The listing builds one solid part. Answer for the finished solid, in the listing's coordinates (mm). A direction names the side the tool comes from. Give positions to 0.01 mm unless a question says otherwise; leave off trailing zeros. Write each loop counter-clockwise with the first axis right and the second up, starting at its lowest first coordinate (ties: lowest second). Pieces come first, ordered by that corner, then holes. Notation, with made-up numbers: M 17,38.5 L 72,38.5 A13 cw 72,62.5 Z; hole C -6.5,-1.5 d5. An arc over 180 degrees is marked long. Answer as a JSON object with one key per item and string values.
Autodesk Inventor part; units mm, degrees
ref_plane "YZ Plane" through (0, 0, 0) normal (1, 0, 0) x (0, 1, 0)
ref_plane "XZ Plane" through (0, 0, 0) normal (0, 1, 0) x (-1, 0, 0)
ref_plane "XY Plane" through (0, 0, 0) normal (0, 0, 1) x (1, 0, 0)
sketch "Sketch1" plane through (0, 0, 0) normal (0, 0, 1) x (1, 0, 0)
  line L0 (-13, 23) -> (13, 23)
  line L1 (15, 21) -> (15, -23)
  line L2 (15, -23) -> (-15, -23)
  line L3 (-15, -23) -> (-15, 21)
  line L4 (-15, 23) -> (15, -23) construction
  line L5 (15, 23) -> (-15, -23) construction
  line L6 (-13, 23) -> (-15, 21)
  line L7 (13, 23) -> (15, 21)
  circle A0 centre (-10, 18.5) radius 1.6
  circle A1 centre (10, 18.5) radius 1.6
  line L8 (10, 18.5) -> (-10, 18.5) construction
  point P0 (0, 0)
  point P1 (0, 18.5)
  point P2 (0, 0)
  dimension "d0" = 30
  dimension "d1" = 46
  dimension "d2" = 2
  dimension "d3" = 2
  dimension "d4" = 2
  dimension "d5" = 2
  dimension "d6" = 3.2
  dimension "d7" = 20
  dimension "d8" = 4.5
extrude "Extrusion1" add sketch "Sketch1" along normal blind 1.6
sketch "Sketch2" plane through (0, 0, 1.6) normal (0, 0, 1) x (1, 0, 0)
  line L0 (10.9, -19) -> (9.1, -19)
  line L1 (9.1, -19) -> (9.1, -4.2)
  line L2 (9.1, -4.2) -> (10.9, -4.2)
  line L3 (10.9, -4.2) -> (10.9, -19)
  line L4 (0.9, -19) -> (-0.9, -19)
  line L5 (-0.9, -19) -> (-0.9, -4.2)
  line L6 (-0.9, -4.2) -> (0.9, -4.2)
  line L7 (0.9, -4.2) -> (0.9, -19)
  line L8 (-9.1, -19) -> (-10.9, -19)
  line L9 (-10.9, -19) -> (-10.9, -4.2)
  line L10 (-10.9, -4.2) -> (-9.1, -4.2)
  line L11 (-9.1, -4.2) -> (-9.1, -19)
  line L12 (-15, 21) -> (-15, -23)
  line L13 (-15, -23) -> (15, -23)
  line L14 (15, -23) -> (15, 21)
  line L15 (15, 21) -> (13, 23)
  line L16 (13, 23) -> (-13, 23)
  line L17 (-13, 23) -> (-15, 21)
  circle A0 centre (10, 18.5) radius 1.6
  circle A1 centre (-10, 18.5) radius 1.6
  line L18 (-0.9, -4.2) -> (0.9, -19) construction
  line L19 (0.9, -4.2) -> (-0.9, -19) construction
  line L20 (10.9, -4.2) -> (9.1, -19) construction
  line L21 (9.1, -4.2) -> (10.9, -19) construction
  line L22 (-10.9, -4.2) -> (-9.1, -19) construction
  line L23 (-9.1, -4.2) -> (-10.9, -19) construction
  point P0 (0, 0)
  point P1 (0, -11.6)
  dimension "d11" = 1.8
  dimension "d12" = 14.8
  dimension "d13" = 4
  dimension "d14" = 8.2
  dimension "d15" = 8.2
extrude "Extrusion2" add sketch "Sketch2" along normal blind 18.2 contours L0 L1 L2 L3 | L4 L5 L6 L7 | L8 L9 L10 L11
fillet "Fillet1" radius 1 6 edges at (-10, -19, 19.8) (-10, -4.2, 19.8) (0, -4.2, 19.8) (0, -19, 19.8) (10, -19, 19.8) (10, -4.2, 19.8)
sketch "Sketch3" plane through (9.1, -19, 1.6) normal (-1, 0, 0) x (0, 0, 1)
  arc A0 (18.2, 13.8) -> (17.2, 14.8) centre (17.2, 13.8) ccw
  line L0 (0, 14.8) -> (17.2, 14.8)
  line L1 (0, 0) -> (0, 14.8)
  line L2 (0, 0) -> (17.2, 0)
  arc A1 (17.2, 0) -> (18.2, 1) centre (17.2, 1) ccw
  line L3 (18.2, 13.8) -> (18.2, 1)
  line L4 (0, 0) -> (0, 14.8)
  line L5 (10, 13.4) -> (0, 13.4)
  line L6 (0, 13.4) -> (0, 1.4)
  line L7 (0, 1.4) -> (10, 1.4)
  line L8 (10, 1.4) -> (10, 13.4)
  line L9 (10, 13.4) -> (0, 1.4) construction
  line L10 (0, 13.4) -> (10, 1.4) construction
  point P0 (-1.6, 19)
  point P1 (5, 7.4)
  point P2 (5, 7.4)
  point P3 (18.2, 7.4)
  point P4 (0, 13.4)
  point P5 (0, 1.4)
  dimension "d19" = 10
  dimension "d20" = 12
extrude "Extrusion3" add sketch "Sketch3" along normal up to surface (18.2 mm away) contours L5 L8 L7 L1
sketch "Sketch4" plane through (0, 0, 1.6) normal (0, 0, 1) x (1, 0, 0)
  circle A0 centre (-10, 18.5) radius 1.6
  circle A1 centre (10, 18.5) radius 1.6
  line L0 (-15, 21) -> (-15, -23)
  line L1 (-15, -23) -> (15, -23)
  line L2 (15, -23) -> (15, 21)
  line L3 (15, 21) -> (13, 23)
  line L4 (13, 23) -> (-13, 23)
  line L5 (-13, 23) -> (-15, 21)
  line L6 (-0.9, -17.6) -> (-9.1, -17.6)
  line L7 (-9.1, -17.6) -> (-9.1, -19)
  line L8 (-9.1, -19) -> (-10.9, -19)
  line L9 (-10.9, -19) -> (-10.9, -4.2)
  line L10 (-10.9, -4.2) -> (-9.1, -4.2)
  line L11 (-9.1, -4.2) -> (-9.1, -5.6)
  line L12 (-9.1, -5.6) -> (-0.9, -5.6)
  line L13 (-0.9, -5.6) -> (-0.9, -4.2)
  line L14 (-0.9, -4.2) -> (0.9, -4.2)
  line L15 (0.9, -4.2) -> (0.9, -5.6)
  line L16 (0.9, -5.6) -> (9.1, -5.6)
  line L17 (9.1, -5.6) -> (9.1, -4.2)
  line L18 (9.1, -4.2) -> (10.9, -4.2)
  line L19 (10.9, -4.2) -> (10.9, -19)
  line L20 (10.9, -19) -> (9.1, -19)
  line L21 (9.1, -19) -> (9.1, -17.6)
  line L22 (9.1, -17.6) -> (0.9, -17.6)
  line L23 (0.9, -17.6) -> (0.9, -19)
  line L24 (0.9, -19) -> (-0.9, -19)
  line L25 (-0.9, -19) -> (-0.9, -17.6)
  line L26 (0.75, 17) -> (-0.75, 17)
  line L27 (-1.25, 16.5) -> (-1.25, 15)
  line L28 (-0.75, 14.5) -> (0.75, 14.5)
  line L29 (1.25, 15) -> (1.25, 16.5)
  line L30 (1.25, 16.5) -> (0.75, 17)
  line L31 (1.25, 15) -> (0.75, 14.5)
  line L32 (-0.75, 14.5) -> (-1.25, 15)
  line L33 (-1.25, 16.5) -> (-0.75, 17)
  line L34 (-3.75, 16.5) -> (-3.25, 17)
  line L35 (-3.75, 16.5) -> (-3.75, 15)
  line L36 (-3.25, 14.5) -> (-3.75, 15)
  line L37 (-1.75, 17) -> (-3.25, 17)
  line L38 (-3.25, 14.5) -> (-1.75, 14.5)
  line L39 (-1.25, 15) -> (-1.75, 14.5)
  line L40 (-1.25, 15) -> (-1.25, 16.5)
  line L41 (-1.25, 16.5) -> (-1.75, 17)
  line L42 (1.25, 16.5) -> (1.75, 17)
  line L43 (1.25, 16.5) -> (1.25, 15)
  line L44 (1.75, 14.5) -> (1.25, 15)
  line L45 (3.25, 17) -> (1.75, 17)
  line L46 (1.75, 14.5) -> (3.25, 14.5)
  line L47 (3.75, 15) -> (3.25, 14.5)
  line L48 (3.75, 15) -> (3.75, 16.5)
  line L49 (3.75, 16.5) -> (3.25, 17)
  line L50 (-1.25, 16.5) -> (-0.75, 17)
  line L51 (-1.25, 16.5) -> (-1.25, 15)
  line L52 (-0.75, 14.5) -> (-1.25, 15)
  line L53 (0.75, 17) -> (-0.75, 17)
  line L54 (-0.75, 14.5) -> (0.75, 14.5)
  line L55 (1.25, 15) -> (0.75, 14.5)
  line L56 (1.25, 15) -> (1.25, 16.5)
  line L57 (1.25, 16.5) -> (0.75, 17)
  point P0 (0, 0)
  point P1 (1.25, 17)
  point P2 (-1.25, 14.5)
  point P3 (-1.25, 17)
  point P4 (1.25, 14.5)
  point P5 (0, 17)
  point P6 (0, 23)
  point P7 (-3.75, 17)
  point P8 (-3.75, 14.5)
  point P9 (-2.5, 17)
  point P10 (-1.25, 17)
  point P11 (-1.25, 14.5)
  point P12 (1.25, 17)
  point P13 (1.25, 14.5)
  point P14 (2.5, 17)
  point P15 (3.75, 17)
  point P16 (3.75, 14.5)
  point P17 (-1.25, 17)
  point P18 (-1.25, 14.5)
  point P19 (0, 17)
  point P20 (1.25, 17)
  point P21 (1.25, 14.5)
  dimension "d23" = 2.5
  dimension "d24" = 2.5
  dimension "d25" = 0.5
  dimension "d26" = 0.5
  dimension "d27" = 0.5
  dimension "d28" = 0.5
  dimension "d29" = 0.5
  dimension "d30" = 0.5
  dimension "d31" = 0.5
  dimension "d32" = 0.5
  dimension "d33" = 6
  dimension "d36" = 2.5
  dimension "d39" = 2.5
extrude "Extrusion4" add sketch "Sketch4" along normal blind 2 contours L30 L29 L31 L28 L32 L27 L33 L26 | L42 L45 L49 L48 L47 L46 L44 L29 | L27 L39 L38 L36 L35 L34 L37 L41
sketch "Sketch5" plane through (0, 0, 3.6) normal (0, 0, 1) x (1, 0, 0)
  line L0 (1.25, 16.5) -> (0.75, 17)
  line L1 (0.75, 17) -> (-0.75, 17)
  line L2 (-0.75, 17) -> (-1.25, 16.5)
  line L3 (-1.25, 16.5) -> (-1.75, 17)
  line L4 (-1.75, 17) -> (-3.25, 17)
  line L5 (-3.25, 17) -> (-3.75, 16.5)
  line L6 (-3.75, 16.5) -> (-3.75, 15)
  line L7 (-3.75, 15) -> (-3.25, 14.5)
  line L8 (-3.25, 14.5) -> (-1.75, 14.5)
  line L9 (-1.75, 14.5) -> (-1.25, 15)
  line L10 (-1.25, 15) -> (-0.75, 14.5)
  line L11 (-0.75, 14.5) -> (0.75, 14.5)
  line L12 (0.75, 14.5) -> (1.25, 15)
  line L13 (1.25, 15) -> (1.75, 14.5)
  line L14 (1.75, 14.5) -> (3.25, 14.5)
  line L15 (3.25, 14.5) -> (3.75, 15)
  line L16 (3.75, 15) -> (3.75, 16.5)
  line L17 (3.75, 16.5) -> (3.25, 17)
  line L18 (3.25, 17) -> (1.75, 17)
  line L19 (1.75, 17) -> (1.25, 16.5)
  line L20 (-3.75, 16.5) -> (-3.75, 15)
  line L21 (2.75, 15.5) -> (2.25, 15.5)
  line L22 (2.25, 15.5) -> (2.25, 16)
  line L23 (2.25, 16) -> (2.75, 16)
  line L24 (2.75, 16) -> (2.75, 15.5)
  line L25 (2.75, 15.5) -> (2.25, 16) construction
  line L26 (2.25, 15.5) -> (2.75, 16) construction
  line L27 (0.25, 15.5) -> (-0.25, 15.5)
  line L28 (-0.25, 15.5) -> (-0.25, 16)
  line L29 (-0.25, 16) -> (0.25, 16)
  line L30 (0.25, 16) -> (0.25, 15.5)
  line L31 (0.25, 15.5) -> (-0.25, 16) construction
  line L32 (-0.25, 15.5) -> (0.25, 16) construction
  line L33 (-2.25, 15.5) -> (-2.75, 15.5)
  line L34 (-2.75, 15.5) -> (-2.75, 16)
  line L35 (-2.75, 16) -> (-2.25, 16)
  line L36 (-2.25, 16) -> (-2.25, 15.5)
  line L37 (-2.25, 15.5) -> (-2.75, 16) construction
  line L38 (-2.75, 15.5) -> (-2.25, 16) construction
  point P0 (0, 0)
  point P1 (2.5, 15.75)
  point P2 (0, 15.75)
  point P3 (-2.5, 15.75)
  point P4 (2.5, 14.5)
  point P5 (0, 14.5)
  point P6 (-2.5, 14.5)
  point P7 (-3.75, 15.75)
  point P8 (-3.75, 15.75)
  point P9 (3.75, 15.75)
  dimension "d44" = 0.5
  dimension "d45" = 0.5
  dimension "d46" = 0.5
  dimension "d47" = 0.5
  dimension "d48" = 0.5
  dimension "d49" = 0.5
extrude "Extrusion5" add sketch "Sketch5" along normal blind 6 contours L21 L22 L23 L24 | L27 L28 L29 L30 | L33 L34 L35 L36
sketch "Sketch6" plane through (9.1, -17.6, 11.6) normal (0, 0, 1) x (1, 0, 0)
  line L0 (-8.2, 0) -> (-8.2, 12)
  line L1 (0, 0) -> (-8.2, 0)
  line L2 (0, 12) -> (0, 0)
  line L3 (0, 12) -> (-8.2, 12)
  line L4 (-10, 12) -> (-10, 0)
  line L5 (-10, 12) -> (-18.2, 12)
  line L6 (-18.2, 0) -> (-18.2, 12)
  line L7 (-10, 0) -> (-18.2, 0)
  line L8 (-7.2, 1) -> (-7.2, 11)
  line L9 (-7.2, 11) -> (-1, 11)
  line L10 (-1, 11) -> (-1, 1)
  line L11 (-1, 1) -> (-7.2, 1)
  line L12 (-17.2, 1) -> (-17.2, 11)
  line L13 (-17.2, 11) -> (-11, 11)
  line L14 (-11, 11) -> (-11, 1)
  line L15 (-11, 1) -> (-17.2, 1)
  point P0 (-9.1, 17.6)
  dimension "d52" = 1
  dimension "d53" = 1
extrude "Extrusion6" add sketch "Sketch6" along normal blind 3 contours L8 L9 L10 L11 | L12 L13 L14 L15
fillet "Fillet2" radius 2 4 edges at (5, -6.6, 14.6) (5, -16.6, 14.6) (-5, -6.6, 14.6) (-5, -16.6, 14.6)
fillet "Fillet3" radius 0.5 20 edges at (8.1, -6.6, 12.1) (8.1, -11.6, 14.6) (8.1, -16.0142, 14.0142) (8.1, -16.6, 12.1) (8.1, -7.1858, 14.0142) (1.9, -11.6, 14.6) (1.9, -16.0142, 14.0142) (1.9, -16.6, 12.1) (1.9, -6.6, 12.1) (1.9, -7.1858, 14.0142) (-1.9, -6.6, 12.1) (-1.9, -11.6, 14.6) (-1.9, -16.0142, 14.0142) (-1.9, -16.6, 12.1) (-1.9, -7.1858, 14.0142) (-8.1, -11.6, 14.6) (-8.1, -16.0142, 14.0142) (-8.1, -16.6, 12.1) (-8.1, -6.6, 12.1) (-8.1, -7.1858, 14.0142)
equation "\"d3\" = d2"
equation "\"d4\" = d2"
equation "\"d5\" = d4"
equation "\"d15\" = d14"
properties part number "current sensor" material "ABS Plastic"
1. Consider line 1 along X through (y, z) = (-10, 13.5); line 2 along Y through (x, z) = (-10, 1.2); line 3 along Z through (x, y) = (13, -6.5). Determine where each line is inside the solid, lowest interval first.
Verdict:
{"line 1": "x = -10.9 to -9.1, -8.1 to -1.9, -0.9 to 0.9, 1.9 to 8.1, 9.1 to 10.9", "line 2": "y = -23 to 16.9, 20.1 to 23", "line 3": "z = 0 to 1.6"}
2. Flat-ended cylindrical pins translate along their axes: pin 1 (3 mm diameter, centred on x = 6.5, z = 4, fed in from -Y); pin 2 (7.5 mm diameter, centred on y = -10, z = 14.5, fed in from -X); pin 3 (1 mm diameter, centred on x = -12, z = 8.5, fed in from +Y); pin 4 (1.6 mm diameter, centred on x = 0, z = 2.5, fed in from -Y). Find the tip coordinate at first contact, or state that the pin passes through.
Verdict:
{"pin 1": "stops at y = -17.6", "pin 2": "stops at x = -10.9", "pin 3": "passes through", "pin 4": "stops at y = -19"}
3. A cutting plane is placed at C-C, the plane y = 18.5. Give the vertices of the cut face in (x, z), plus the area to 3 significant figures.
Verdict:
{"outline": "M -15,0 L -11.6,0 L -11.6,1.6 L -15,1.6 Z; M -8.4,0 L 8.4,0 L 8.4,1.6 L -8.4,1.6 Z; M 11.6,0 L 15,0 L 15,1.6 L 11.6,1.6 Z", "area": "37.8 mm2"}
4. A cutting plane is placed at B-B, the plane x = 10. Give the vertices of the cut face in (y, z).
Verdict:
{"outline": "M -23,0 L 16.9,0 L 16.9,1.6 L -4.2,1.6 L -4.2,18.8 A1 ccw -5.2,19.8 L -18,19.8 A1 ccw -19,18.8 L -19,1.6 L -23,1.6 Z; M 20.1,0 L 23,0 L 23,1.6 L 20.1,1.6 Z"}
5. The mould has two halves that part along X. Classify faces 1 (the flat face through (-5, -17.6, 7)), 2 (the flat face through (10, -4.2, 10)), 3 (the flat face through (14, 22, 1)): released by +X, released by -X, zero draft, split by the parting line, or undercut.
Verdict:
{"face 1": "undercut", "face 2": "zero draft", "face 3": "released by +X"}
6. A cutting plane is placed at A-A, the plane z = 17.5. Give the vertices of the cut face in (x, y), plus the area to 3 significant figures.
Verdict:
{"outline": "M -10.9,-19 L -9.1,-19 L -9.1,-4.2 L -10.9,-4.2 Z; M -0.9,-19 L 0.9,-19 L 0.9,-4.2 L -0.9,-4.2 Z; M 9.1,-19 L 10.9,-19 L 10.9,-4.2 L 9.1,-4.2 Z", "area": "79.9 mm2"}
7. For faces 4 (the cylindrical face through (-5.04, -16.03, 14)), 5 (the flat face through (-5, -6.6, 12)), 6 (the flat face through (10, -19, 10)), determine the directions among +Z, -Z, +X, -X, +Y, -Y from which every point of the face is accessible in a straight line to the end or side of a thin tool.
Verdict:
{"face 4": "+Z, -Y", "face 5": "+Z, +Y", "face 6": "+Z, +X, -X, -Y"}
8. A cutting plane is placed at D-D, the plane z = 5.75. Count the separate pieces of the cut face and the enclosed holes in it, plus the area to 3 significant figures.
Verdict:
{"separate pieces": "4", "enclosed holes": "0", "area": "277 mm2"}
